from build123d import *

# Parameters (mm, degrees)
CHAPAINFERIOR_DEPTH   = 4
CORTE_EXTRUS_O1_DEPTH = 398.008816023


with BuildPart() as part:
    # Chapa inferior → ChapaInferior (new, symmetric)
    with BuildSketch(Plane(origin=(0, 0, 0), x_dir=(1, 0, 0), z_dir=(0, 1, 0))):
        with BuildLine():
            Line((-160, 300), (160, 300))
            ThreePointArc((160, 300), (230.710678119, 270.710678119), (260, 200))
            Line((260, 200), (260, -200))
            ThreePointArc((260, -200), (230.710678119, -270.710678119), (160, -300))
            Line((160, -300), (-160, -300))
            ThreePointArc((-160, -300), (-230.710678119, -270.710678119), (-260, -200))
            Line((-260, -200), (-260, 200))
            ThreePointArc((-260, 200), (-230.710678119, 270.710678119), (-160, 300))
        make_face()
    extrude(amount=CHAPAINFERIOR_DEPTH, both=True)

    # Esboço2 → Corte-extrusão1 (cut, through all)
    with BuildSketch(Plane(origin=(0, 0, 0), x_dir=(1, 0, 0), z_dir=(0, 1, 0))):
        with BuildLine():
            Line((-150, -251), (150, -251))
            ThreePointArc((150, -251), (162, -263), (150, -275))
            Line((150, -275), (-150, -275))
            ThreePointArc((-150, -275), (-162, -263), (-150, -251))
        make_face()
    extrude(amount=CORTE_EXTRUS_O1_DEPTH, mode=Mode.SUBTRACT)


solid = part.part
Geometry: final body of the model. Coordinates: model frame, mm. A direction names the side the tool comes from. Round coordinates to 2 decimals unless told otherwise and drop trailing zeros. Order: outer loops, then holes, each group sorted by start corner. A loop starts at its lowest first (then second) coordinate and runs counter-clockwise, first axis right, second up.
Q1. Section B-B, the plane x = 7.5. Output: boundary loops of the cut face in (y, z).
Result sheet:
outline: (-4, -300) - (4, -300) - (4, 251) - (0, 251) - (0, 275) - (4, 275) - (4, 300) - (-4, 300) - close
Q2. Section A-A, the plane y = 1.75. Output: boundary loops of the cut face in (x, z), and give its area (3 significant figures).
Result sheet:
outline: (-260, -200) arc R100 ccw to (-160, -300) - (160, -300) arc R100 ccw to (260, -200) - (260, 200) arc R100 ccw to (160, 300) - (-160, 300) arc R100 ccw to (-260, 200) - close; hole (-150, 251) - (150, 251) arc R12 ccw to (150, 275) - (-150, 275) arc R12 ccw to start
area: 296,000 mm2
Q3. Material intervals for probe 1 along Z at (x, y) = (47, 2.5); probe 2 along Z at (x, y) = (-191.5, 1.25); probe 3 along X at (y, z) = (-1.5, -230), sorted ascending.
Result sheet:
probe 1: z = -300 to 251, 275 to 300
probe 2: z = -294.91 to 294.91
probe 3: x = -255.39 to 255.39
Q4. Section C-C, the plane z = 263. Output: boundary loops of the cut face in (x, y).
Result sheet:
outline: (-237.66, -4) - (237.66, -4) - (237.66, 4) - (162, 4) - (162, 0) - (-162, 0) - (-162, 4) - (-237.66, 4) - close
Q5. Pin query (flat end, axial travel): pin 1 (12 mm diameter, centred on x = -22.5, z = 257.5, fed in from +Y). Return the tip coordinate at first contact, or that it passes through.
Result sheet:
pin 1: stops at y = 0
Q6. Access query for faces 1 (the face through (-162, 2, 263)), 2 (the face through (-231.484, 0.056, -269.929)). Directions: +Z, -Z, +X, -X, +Y, -Y. A direction counts if a zero-diameter tool reaches every point of the face in a straight line with its end or side. Return the directions, or none.
Result sheet:
face 1: +Y
face 2: -Z, -X, +Y, -Y
Q7. Section D-D, the plane x = -198.5. Output: boundary loops of the cut face in (y, z), and give its area (3 significant figures).
Result sheet:
outline: (-4, -292.29) - (4, -292.29) - (4, 292.29) - (-4, 292.29) - close
area: 4,680 mm2
Q8. Mould query, pull axis Z, two halves, no side actions, for faces 3 (the face through (-229.929, 0.056, 271.484)), 4 (the face through (162, 2, 263)), 5 (the face through (4, 4, -4)). Classes: released by +Z, released by -Z, zero draft, split by the parting line, or undercut.
Result sheet:
face 3: released by +Z
face 4: undercut
face 5: zero draft
